Autodesk Fusion 360 part; units mm, degrees
sketch "Sketch1" plane through (0, 0, 0) normal (0, 0, 1) x (1, 0, 0)
  line L0 (30, 30) -> (-30, 30)
  line L1 (-30, 30) -> (-30, -30)
  line L2 (-30, -30) -> (30, -30)
  line L3 (30, -30) -> (30, 30)
  line L4 (30, 30) -> (-30, -30) construction
  line L5 (-30, 30) -> (30, -30) construction
  circle A0 centre (-30, 30) radius 2.8
  circle A1 centre (30, 30) radius 2.8
  circle A2 centre (-30, -30) radius 2.8
  circle A3 centre (30, -30) radius 2.8
  line L6 (50, 50) -> (-50, 50)
  line L7 (-50, 50) -> (-50, -50)
  line L8 (-50, -50) -> (50, -50)
  line L9 (50, -50) -> (50, 50)
  line L10 (50, 50) -> (-50, -50) construction
  line L11 (-50, 50) -> (50, -50) construction
  line L12 (50, 50) -> (-50, 50)
  line L13 (-50, 50) -> (-50, 60)
  line L14 (-50, 60) -> (50, 60)
  line L15 (50, 60) -> (50, 50)
  line L16 (50, -50) -> (-50, -50)
  line L17 (-50, -50) -> (-50, -60)
  line L18 (-50, -60) -> (50, -60)
  line L19 (50, -60) -> (50, -50)
  circle A4 centre (-30, 30) radius 2
  circle A5 centre (30, 30) radius 2
  circle A6 centre (-30, -30) radius 2
  circle A7 centre (30, -30) radius 2
  dimension "d1" = 60
  dimension "d2" = 60
  dimension "d3" = 5.6
  dimension "d6" = 60
  dimension "d7" = -60
  dimension "d8" = 100
  dimension "d9" = 100
  dimension "d12" = 100
  dimension "d13" = 10
  dimension "d14" = 100
  dimension "d15" = 10
  dimension "d26" = 4
extrude "Extrude1" add sketch "Sketch1" along normal blind 10 contours L0 L1 L2 L3 A0 A1 A2 A3 | L6 L7 L8 L9 L12 L16 makes body 1
extrude "Extrude2" add sketch "Sketch1" along normal blind 110 contours L6 L12 L13 L14 L15 | L8 L16 L17 L18 L19 bodies 1
sketch "Sketch2" plane through (0, 0, 110) normal (0, 0, 1) x (1, 0, 0)
  line L0 (50, 60) -> (-50, 60)
  line L1 (-50, 60) -> (-50, 50)
  line L2 (-50, 50) -> (50, 50)
  line L3 (50, 50) -> (50, 60)
  circle A0 centre (-40, 55) radius 2.8
  line L4 (-50, 55) -> (50, 55)
  circle A1 centre (0, 55) radius 2.8
  circle A2 centre (40, 55) radius 2.8
  circle A3 centre (-40, -55) radius 2.8
  circle A4 centre (0, -55) radius 2.8
  circle A5 centre (40, -55) radius 2.8
  line L5 (-50, 60) -> (50, 60)
  line L6 (50, 60) -> (50, -60)
  line L7 (50, -60) -> (-50, -60)
  line L8 (-50, -60) -> (-50, 60)
  circle A6 centre (-40, 55) radius 2.25
  circle A7 centre (0, 55) radius 2.25
  circle A8 centre (40, 55) radius 2.25
  circle A9 centre (-40, -55) radius 2.25
  circle A10 centre (0, -55) radius 2.25
  circle A11 centre (40, -55) radius 2.25
  dimension "d18" = 5.6
  dimension "d19" = 10
  dimension "d22" = 40
  dimension "d23" = -110
  dimension "d30" = 120
  dimension "d31" = 100
  dimension "d32" = 4.5
extrude "Extrude3" cut sketch "Sketch2" against normal blind 8.1 contours L4 A2 A8 | L4 A2 A8 | A0 L4 A6 | A0 L4 A6 | L4 A8 | L4 A8 | L4 A6 | L4 A6 | L4 A1 A7 | L4 A1 A7 | L4 A7 | L4 A7 | A3 | A4 | A5 | A9 | A10 | A11 bodies 1
extrude "Extrude4" add sketch "Sketch1" against normal blind 1.9 from surface at 10 contours L0 L1 A0 A4 | L0 L1 A0 A4 | L0 L3 A1 A5 | L0 L3 A1 A5 | L1 L2 A2 A6 | L1 L2 A2 A6 | L2 L3 A3 A7 | L2 L3 A3 A7 bodies 1
extrude "Extrude5" add sketch "Sketch2" along normal blind 12 separate body contours L0 L1 L3 A0 L4 A1 A2 L5 L6 L8 | L1 L2 L3 A0 L4 A1 A2 L6 L8 | L2 L6 L7 L8 | L4 A2 A8 | L4 A2 A8 | A0 L4 A6 | A0 L4 A6 | L4 A1 A7 | L4 A1 A7 | A3 | A4 | A5 makes body 2
chamfer "Chamfer1" distance 5 angle 45 4 edges at (-50, 0, 0) (0, 60, 0) (50, 0, 0) (0, -60, 0) on bodies 1
hidden bodies 1
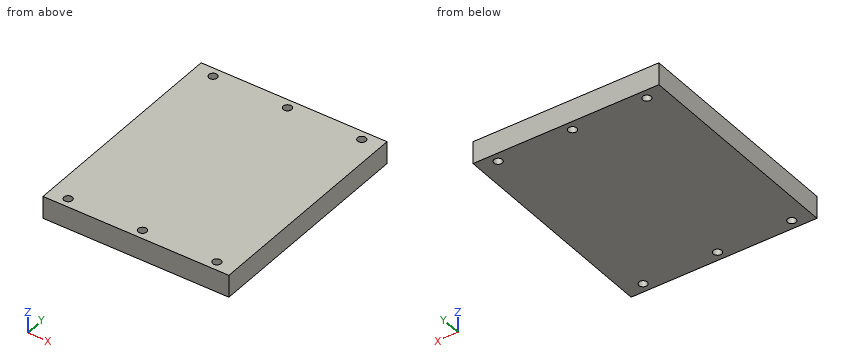
Can you work these out from the model? Positions are in its coordinate system, mm. Round coordinates to 2 decimals unless told otherwise and drop trailing zeros. Order: outer loops, then holes, each group sorted by start corner. A loop starts at its lowest first (then second) coordinate and runs counter-clockwise, first axis right, second up. Notation, with made-up numbers: (26, 15) - (74, 15) arc R19 cw to (74, 51) - close; hole circle Ø11 at (-10.5, 67). An arc over 180 degrees is marked (long way). Answer in a Markdown table with one row per item.
(1) For P1, Ø6, axis at x = 0, y = 55, coming from the +Z side, with a flat end and sliding along its axis, tell me the tip position at first contact or that it passes through.
From the geometry:
| item | result |
|---|---|
| P1 | stops at z = 122 |
(2) Suppose I cut it at B-B, the plane y = -55. Please give me the cut outline in (x, z), plus the area to 3 significant figures.
From the geometry:
| item | result |
|---|---|
| outline | (-50, 110) - (-42.25, 110) - (-42.25, 122) - (-50, 122) - close; (-37.75, 110) - (-2.25, 110) - (-2.25, 122) - (-37.75, 122) - close; (2.25, 110) - (37.75, 110) - (37.75, 122) - (2.25, 122) - close; (42.25, 110) - (50, 110) - (50, 122) - (42.25, 122) - close |
| area | 1,040 mm2 |
(3) Please list where these lines run through material, in increasing order: L1, parallel to X at y = 55, z = 115.5; L2, parallel to Y at x = -40, z = 113; L3, parallel to Y at x = -41, z = 114.5. Write a range as from..to.
From the geometry:
| item | result |
|---|---|
| L1 | x = -50..-42.25, -37.75..-2.25, 2.25..37.75, 42.25..50 |
| L2 | y = -60..-57.25, -52.75..52.75, 57.25..60 |
| L3 | y = -60..-57.02, -52.98..52.98, 57.02..60 |
(4) Suppose I cut it at A-A, the plane x = 0. Please give me the cut outline in (y, z).
From the geometry:
| item | result |
|---|---|
| outline | (-60, 110) - (-57.25, 110) - (-57.25, 122) - (-60, 122) - close; (-52.75, 110) - (52.75, 110) - (52.75, 122) - (-52.75, 122) - close; (57.25, 110) - (60, 110) - (60, 122) - (57.25, 122) - close |
